Here's how the part is built. I have some questions about the finished solid (model axes, mm). Round coordinates to 2 decimals unless told otherwise and drop trailing zeros. Order: outer loops, then holes, each group sorted by start corner. A loop starts at its lowest first (then second) coordinate and runs counter-clockwise, first axis right, second up. Notation, with made-up numbers: (80, 63) - (85, 63) arc R20 ccw to (85, 79) - close; hole circle Ø7 at (-39, -24.75). An arc over 180 degrees is marked (long way). Answer as a JSON object with one key per item and string values.
```python
from build123d import *

# Parameters (mm, degrees)
F0_W     = 177.8
F0_H     = 159.512
F1_DEPTH = 12.7
F3_DEPTH = 12.701


with BuildPart() as f1:
    # F0 (on Top) → F1 (new body)
    with BuildSketch(Plane.XY):
        with Locations((88.9, 79.756)):
            Rectangle(F0_W, F0_H)
    extrude(amount=F1_DEPTH)

    # F2 (on face) → F3 (cut, through all)
    with BuildSketch(Plane.XY.offset(12.7)):
        with BuildLine():
            Line((139.7, 159.512), (38.1, 159.512))
            Line((38.1, 159.512), (38.1, 146.812))
            ThreePointArc((38.1, 146.812), (41.819744, 137.831744), (50.8, 134.112))
            Line((50.8, 134.112), (88.9, 134.112))
            Line((88.9, 134.112), (127, 134.112))
            ThreePointArc((127, 134.112), (135.980256, 137.831744), (139.7, 146.812))
            Line((139.7, 146.812), (139.7, 159.512))
        make_face()
    extrude(amount=-F3_DEPTH, mode=Mode.SUBTRACT)


solid = f1.part
```
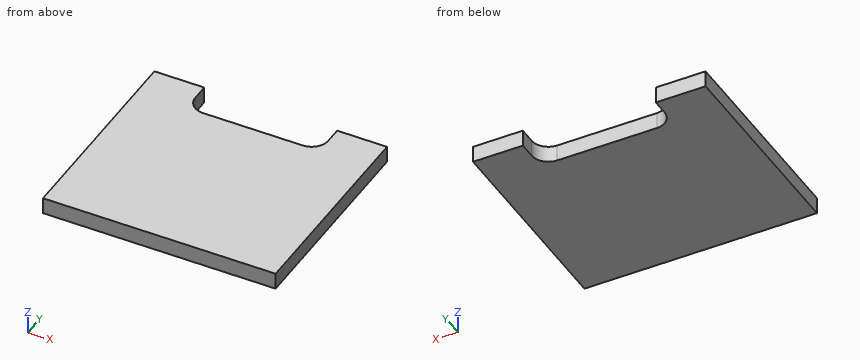
1. If I drill on L1, parallel to Y at x = 92, z = 3; L2, parallel to Y at x = 137, z = 2, over which ranges is the centre line in solid material (lowest first)? Write a range as [from, to].
Responses:
{"L1": "[0, 134.11]", "L2": "[0, 138.98]"}
2. Imagine slicing it at B-B (x = 96.5). List the corners of the cut face in (y, z) for me.
Responses:
{"outline": "(0, 0) - (134.11, 0) - (134.11, 12.7) - (0, 12.7) - close"}
3. For P1, Ø6.5, axis at x = 73, z = 9.5, coming from the +Y side, with a flat end and sliding along its axis, tell me the tip position at first contact or that it passes through.
Responses:
{"P1": "y = 134.11"}
4. Imagine slicing it at C-C (x = 132). List the corners of the cut face in (y, z) for me.
Responses:
{"outline": "(0, 0) - (135.14, 0) - (135.14, 12.7) - (0, 12.7) - close"}
5. Imagine slicing it at A-A (z = 3). List the corners of the cut face in (x, y) for me, plus the area to 3 significant figures.
Responses:
{"outline": "(0, 0) - (177.8, 0) - (177.8, 159.51) - (139.7, 159.51) - (139.7, 146.81) arc R12.7 cw to (127, 134.11) - (50.8, 134.11) arc R12.7 cw to (38.1, 146.81) - (38.1, 159.51) - (0, 159.51) - close", "area": "25,800 mm2"}
